Source: CAD feature listing. Evaluate the final solid. Frame: model axes, mm. Face numbers are marked on the shaded views. Round coordinates to 2 decimals unless told otherwise and drop trailing zeros. Order: outer loops, then holes, each group sorted by start corner. A loop starts at its lowest first (then second) coordinate and runs counter-clockwise, first axis right, second up. Notation, with made-up numbers: M 54.25,-11.5 L 68.25,-11.5 A24 cw 68.25,9.5 Z; hole C -20.75,56 d9. An arc over 180 degrees is marked long. Use CSV: the item, a comma, the result in double quotes. Start each with the question number.
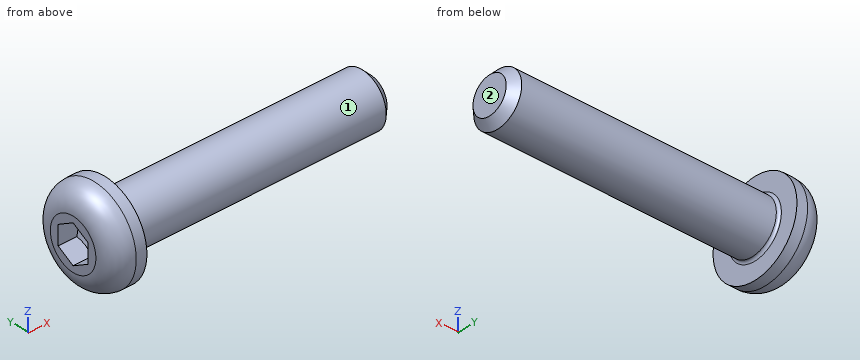
Autodesk Inventor part; units mm, degrees
ref_plane "Work Plane1" through (29, 0, 0) normal (0, -1, 0) x (1, 0, 0)
ref_plane "YZ Plane" through (0, 0, 0) normal (1, 0, 0) x (0, 1, 0)
ref_plane "XZ Plane" through (0, 0, 0) normal (0, 1, 0) x (-1, 0, 0)
sketch "Sketch1" plane through (0, 0, 0) normal (0, 0, 1) x (1, 0, 0)
  line L0 (-0.0833, 0) -> (10, 0)
  line L1 (10, 0) -> (10, 1)
  line L2 (10, 1) -> (7, 1)
  line L3 (7, 1) -> (6.6932, 1)
  line L4 (6.6932, 1) -> (0, 1)
  line L5 (0, 1) -> (0, 1.75)
  line L6 (0, 1.75) -> (-1.2, 1.75)
  line L7 (-1.2, 1.75) -> (-1.2, 0.7217)
  line L8 (-1.2, 0.7217) -> (-0.5, 0.7217)
  line L9 (-0.5, 0.7217) -> (-0.0833, 0)
  line L10 (-3.44, 0) -> (12.24, 0)
  line L11 (0, -0.35) -> (0, 2.1)
  line L12 (7, 1) -> (0, 1) construction
  dimension "d1" = 3
  dimension "d2" = 0.3068
  dimension "d3" = 1.2
  dimension "d4" = 0.7
  dimension "d5" = 60
  dimension "d6" = 2
  dimension "d7" = 2
  dimension "d8" = 1.4434
  dimension "d9" = 3.5
  dimension "d26" = 10
revolve "Body" add sketch "Sketch1" angle 360 about axis through (-0.0833, 0, 0) along (1, 0, 0)
sketch "Sketch2" plane through (-1.2, 0, 0) normal (-1, 0, 0) x (0, 0, 1)
  circle A0 centre (0, 0) radius 0.7217
  line L0 (0, -2.45) -> (0, 2.45)
  line L1 (-2.45, 0) -> (2.45, 0)
  line L2 (0.7217, 0) -> (0.3608, -0.625)
  line L3 (0.3608, -0.625) -> (-0.3608, -0.625)
  line L4 (-0.3608, -0.625) -> (-0.7217, 0)
  line L5 (-0.7217, 0) -> (-0.3608, 0.625)
  line L6 (-0.3608, 0.625) -> (0.3608, 0.625)
  line L7 (0.3608, 0.625) -> (0.7217, 0)
extrude "Slot" add sketch "Sketch2" against normal up to next contours L7 A0 | A0 L2 | L6 L0 A0 | A0 L0 L3 | L0 L6 A0 | A0 L3 L0 | L4 A0 | A0 L5
fillet "Fillet1" radius 0.8 1 edges at (-1.2, -1.75, 0)
chamfer "Chamfer1" distance 0.3067 distance2 0.3067 1 edges at (10, -1, 0) measured on face at (10, -0.5392, -0.3309)
ref_plane "Work Plane1" through (29, 0, 0) normal (0, -1, 0) x (1, 0, 0)
fillet "Fillet2" radius 0.1 1 edges at (0, -1, 0)
thread "Thread2"
equation "\"d15\" = -0.5 * SPD + 0.5 * GD"
equation "\"d16\" = GUL"
equation "\"GD\" = NND"
equation "\"NLG\" = 6"
equation "\"GEL\" = 4.5"
equation "\"KOD\" = 5.7"
equation "\"KOH\" = 1.65"
equation "\"INTI\" = 1.04"
equation "\"GAL\" = 0.61345 * PTC"
equation "\"GUL\" = 0.61345 * PTC"
equation "\"BDM\" = NND"
equation "\"SW\" = 2"
equation "\"RR\" = 1.45"
equation "\"SPD\" = NND - 1.2269 * PTC"
equation "\"R\" = 0.3"
equation "\"TOA\" = 30deg"
equation "\"GD1\" = THREADDIA - 1.2269 * PTC"
equation "\"THREADDIA\" = 3"
equation "\"PTC\" = 0.5"
equation "\"NND\" = 3"
equation "\"KOH1\" = 0.2"
equation "\"E0\" = 2.303"
properties part number "M2x10 Bolt" material "Stainless Steel"
(1) Section A-A on x = 6.5. Return loops of the section in (y, z), plus the area to 3 significant figures.
(2) Draft query along Z for the marked faces 1 and 2. Return one class per face: pulls with the +Z half, pulls with the -Z half, needs draft (parallel to the pull), parting line crosses it, or undercut.
(3) Contact query for a flat-ended pin moving along its axis: P1, Ø1.5, axis at x = 1, z = 1, coming from the +Y side. Output: stop coordinate, or through.
(4) Line query: line 1 along Y through (x, z) = (7.25, -0.1); line 2 along Y through (x, z) = (7, 0.7). Output: solid intervals per line, ascending.
Results below:
1,outline,"C 0,0 d2"
1,area,"3.14 mm2"
2,face 1,"parting line crosses it"
2,face 2,"needs draft"
3,P1,"stops at y = 0.97"
4,line 1,"y = -0.99 to 0.99"
4,line 2,"y = -0.71 to 0.71"
